from build123d import *

# Parameters (mm, degrees)
BOSS_EXTRUDE1_DEPTH = 30.48
SKETCH2_W           = 3.81
SKETCH2_H           = 10.922
BOSS_EXTRUDE2_DEPTH = 78.74
BOSS_EXTRUDE3_DEPTH = 7.62
SKETCH5_R           = 1.905
CUT_EXTRUDE2_DEPTH  = 8.62
SKETCH6_W           = 30.48
SKETCH6_H           = 62.484
CUT_EXTRUDE3_DEPTH  = 7.35


with BuildPart() as part:
    # Sketch1 → Boss-Extrude1 (new body)
    with BuildSketch(Plane(origin=(0, 0, 0), x_dir=(0, 0, -1), z_dir=(1, 0, 0))):
        Polygon((0, 0), (78.74, 0), (78.74, 10.922), (70.612, 10.922), (70.612, 8.382), (74.422, 8.382), (74.422, 6.35), (4.318, 6.35), (4.318, 8.382), (8.128, 8.382), (8.128, 10.922), (0, 10.922), align=None)
    extrude(amount=BOSS_EXTRUDE1_DEPTH)

    # Sketch2 → Boss-Extrude2 (add)
    with BuildSketch(Plane.XY):
        with Locations((-1.905, 5.461)):
            Rectangle(SKETCH2_W, SKETCH2_H)
    extrude(amount=-BOSS_EXTRUDE2_DEPTH)

    # Sketch4 → Boss-Extrude3 (add)
    with BuildSketch(Plane.XZ):
        with BuildLine():
            Line((21.59, 0), (25.704138816, 7.632415502))
            ThreePointArc((25.704138816, 7.632415502), (28.56149521, 8.89), (30.48, 6.427208148))
            Line((30.48, 6.427208148), (30.48, 0))
            Line((30.48, 0), (21.59, 0))
        make_face()
        with BuildLine():
            Line((-3.81, -78.74), (-3.81, -85.167208148))
            ThreePointArc((-3.81, -85.167208148), (-1.89149521, -87.63), (0.965861184, -86.372415502))
            Line((0.965861184, -86.372415502), (5.08, -78.74))
            Line((5.08, -78.74), (-3.81, -78.74))
        make_face()
    extrude(amount=-BOSS_EXTRUDE3_DEPTH)

    # Sketch5 → Cut-Extrude2 (cut, through all)
    with BuildSketch(Plane(origin=(0, 7.62, 0), x_dir=(1, 0, 0), z_dir=(0, 1, 0))):
        with Locations((-0.508, 82.042)):
            Circle(SKETCH5_R)
        with Locations((27.178, -3.302)):
            Circle(SKETCH5_R)
    extrude(amount=-CUT_EXTRUDE2_DEPTH, mode=Mode.SUBTRACT)

    # Sketch6 → Cut-Extrude3 (cut, through all)
    with BuildSketch(Plane(origin=(0, 6.35, 0), x_dir=(1, 0, 0), z_dir=(0, 1, 0))):
        with Locations((15.24, 39.37)):
            Rectangle(SKETCH6_W, SKETCH6_H)
    extrude(amount=-CUT_EXTRUDE3_DEPTH, mode=Mode.SUBTRACT)


solid = part.part
Verification items for the finished model (mm, model axes). A direction names the side the tool comes from. Coordinates: 2 decimals unless noted, no trailing zeros. Write each loop counter-clockwise with the first axis right and the second up, starting at its lowest first coordinate (ties: lowest second). Pieces come first, ordered by that corner, then holes. Notation, with made-up numbers: M 16,-22 L 41,-22 A31 cw 41,13 Z; hole C 75.25,86 d7. An arc over 180 degrees is marked long. Use a Markdown table: item, result.
Q1. Draft check along Y on faces 4 (the face through (15, 8.382, -6)), 5 (the face through (-0.4, 7.62, -84.2)), 6 (the face through (-1.937, 3.757, -87.618)). Enter one of: +Y half, -Y half, draft (parallel to the pull), parting line (faces both ways), or undercut.
Reply:
| item | result |
|---|---|
| face 4 | undercut |
| face 5 | +Y half |
| face 6 | draft |
Q2. Sectioned sample at B-B, the plane x = 27.5. Record the boundary of the cut face in (y, z), plus the area to 3 significant figures.
Reply:
| item | result |
|---|---|
| outline | M 0,-78.74 L 10.92,-78.74 L 10.92,-70.61 L 8.38,-70.61 L 8.38,-74.42 L 6.35,-74.42 L 6.35,-70.61 L 0,-70.61 Z; M 0,-8.13 L 6.35,-8.13 L 6.35,-4.32 L 8.38,-4.32 L 8.38,-8.13 L 10.92,-8.13 L 10.92,0 L 7.62,0 L 7.62,1.42 L 0,1.42 Z; M 0,5.18 L 7.62,5.18 L 7.62,8.93 L 0,8.93 Z |
| area | 201 mm² |
Q3. Sectioned sample at D-D, the plane z = -46. Record the boundary of the cut face in (x, y).
Reply:
| item | result |
|---|---|
| outline | M -3.81,0 L 0,0 L 0,10.92 L -3.81,10.92 Z |
Q4. Sectioned sample at A-A, the plane x = 12.5. Record the boundary of the cut face in (y, z), plus the area to 3 significant figures.
Reply:
| item | result |
|---|---|
| outline | M 0,-78.74 L 10.92,-78.74 L 10.92,-70.61 L 8.38,-70.61 L 8.38,-74.42 L 6.35,-74.42 L 6.35,-70.61 L 0,-70.61 Z; M 0,-8.13 L 6.35,-8.13 L 6.35,-4.32 L 8.38,-4.32 L 8.38,-8.13 L 10.92,-8.13 L 10.92,0 L 0,0 Z |
| area | 162 mm² |
Q5. Sectioned sample at C-C, the plane y = 10. Record the boundary of the cut face in (x, z), plus the area to 3 significant figures.
Reply:
| item | result |
|---|---|
| outline | M -3.81,-78.74 L 30.48,-78.74 L 30.48,-70.61 L 0,-70.61 L 0,-8.13 L 30.48,-8.13 L 30.48,0 L -3.81,0 Z |
| area | 795 mm² |
Q6. Go/stop test with flat-tipped pins: P1, Ø1.6, axis at x = 11.5, y = 7.5, coming from the -Z side; P2, Ø2, axis at x = 25.5, y = 2, coming from the +Z side; P3, Ø5.5, axis at y = 7.5, z = -47.5, coming from the +X side. Record where each tip stops, or that it passes through.
Reply:
| item | result |
|---|---|
| P1 | stops at z = -78.74 |
| P2 | stops at z = 8.52 |
| P3 | stops at x = 0 |
Q7. Set-up check for faces 1 (the face through (27, 7.62, 6)), 2 (the face through (15, 10, -70.612)), 3 (the face through (15, 7, -4.318)): record each of +Z, -Z, +X, -X, +Y, -Y from which the full face is reachable in a straight line by a thin tool's end or side.
Reply:
| item | result |
|---|---|
| face 1 | +Z, +X, -X, +Y |
| face 2 | +X, +Y, -Y |
| face 3 | +X |
Q8. Thickness scan on line 1 (Z direction, x = 16, y = 2.5); line 2 (Z direction, x = 28, y = 5.5); line 3 (Y direction, x = 21, z = -72). Record the ranges inside material, lowest first.
Reply:
| item | result |
|---|---|
| line 1 | z = -78.74 to -70.61, -8.13 to 0 |
| line 2 | z = -78.74 to -70.61, -8.13 to 1.58, 5.02 to 8.97 |
| line 3 | y = 0 to 6.35, 8.38 to 10.92 |
